Design review of the part shown in the three views and the two pictorial views. Dimensions are in mm from the part's minimum x, y and z. A direction names the side the tool comes from. Round coordinates to 2 decimals unless told otherwise and drop trailing zeros. Order: outer loops, then holes, each group sorted by start corner. A loop starts at its lowest first (then second) coordinate and runs counter-clockwise, first axis right, second up.
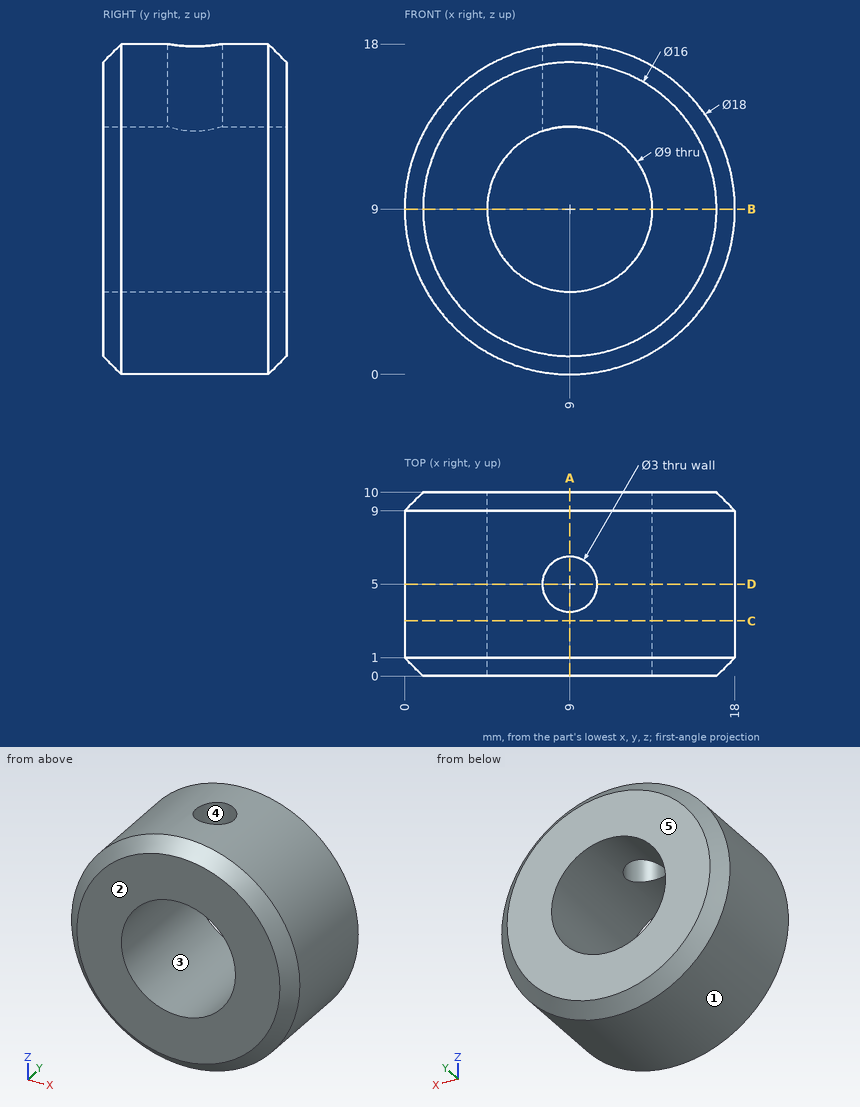
(1) For the marked faces 4 and 5, list the 3-axis set-ups (+Z, -Z, +X, -X, +Y, -Y) from which the entire face can be reached by the end or side of a thin tool; tool diameter is ignored.
Data:
face 4: +Z
face 5: +Z, -Z, +X, -X, +Y
(2) Consider section A-A (x = 9). Write out the cut boundary in (y, z).
Data:
outline: (0, 1) - (1, 0) - (9, 0) - (10, 1) - (10, 4.5) - (0, 4.5) - close; (0, 13.5) - (3.5, 13.5) - (3.5, 18) - (1, 18) - (0, 17) - close; (6.5, 13.5) - (10, 13.5) - (10, 17) - (9, 18) - (6.5, 18) - close
(3) To check wall thickness, follow probe 1 along Z at (x, y) = (9, 2.5); probe 2 along Z at (x, y) = (11, 7.25); probe 3 along X at (y, z) = (6, 6.75). State the ranges of each line that lie inside material, in increasing order.
Data:
probe 1: z = 0 to 4.5, 13.5 to 18
probe 2: z = 0.23 to 4.97, 13.03 to 17.77
probe 3: x = 0.29 to 5.1, 12.9 to 17.71
(4) Consider section C-C (y = 3). Write out the cut boundary in (x, z), and give its area (3 significant figures).
Data:
outline: circle Ø18 at (9, 9); hole circle Ø9 at (9, 9)
area: 191 mm2
(5) Insertion check: pin 1 (3 mm diameter, centred on y = 3, z = 2.5, fed in from -X); pin 2 (4 mm diameter, centred on x = 16, y = 2, fed in from +Z); pin 3 (3 mm diameter, centred on x = 16, y = 2.5, fed in from -Z); pin 4 (5.5 mm diameter, centred on x = 9, z = 9, fed in from -Y). Each pin has a flat end and moves straight along its axis. Give the tip position at first contact, or say it passes through.
Data:
pin 1: stops at x = 1.52
pin 2: stops at z = 16.48
pin 3: stops at z = 1.88
pin 4: passes through
(6) Consider section B-B (z = 9). Write out the cut boundary in (x, y).
Data:
outline: (0, 1) - (1, 0) - (4.5, 0) - (4.5, 10) - (1, 10) - (0, 9) - close; (13.5, 0) - (17, 0) - (18, 1) - (18, 9) - (17, 10) - (13.5, 10) - close
(7) Draft analysis for pull direction X (two halves, no side actions). For the marked faces 1, 2 and 3, state which applies: pulls with the +X half, pulls with the -X half, needs draft (parallel to the pull), parting line crosses it, or undercut.
Data:
face 1: parting line crosses it
face 2: needs draft
face 3: undercut
(8) Consider section D-D (y = 5). Write out the cut boundary in (x, z), and give its area (3 significant figures).
Data:
outline: (7.5, 13.24) - (7.5, 17.87) arc R9 ccw (long way) to (10.5, 17.87) - (10.5, 13.24) arc R4.5 cw (long way) to start
area: 177 mm2
